```python
from build123d import *

# Parameters (mm, degrees)
SKETCH1_W           = 2.032
SKETCH1_H           = 34.925
BOSS_EXTRUDE1_DEPTH = 228.6
CUT_EXTRUDE1_REACH  = 233.261
SKETCH2_R           = 4.7625
LPATTERN1_COUNT     = 24
LPATTERN1_PITCH     = 19.05
FILLET1_R           = 12.7


with BuildPart() as part:
    # Sketch1 → Boss-Extrude1 (new, symmetric)
    with BuildSketch(Plane.XY):
        with Locations((1.016, 17.4625)):
            Rectangle(SKETCH1_W, SKETCH1_H)
    extrude(amount=BOSS_EXTRUDE1_DEPTH, both=True)

    # Sketch2 → Cut-Extrude1 (cut, up to next)
    with BuildSketch(Plane.ZY, mode=Mode.PRIVATE) as cut_extrude1_sk1:
        with Locations((219.075, 17.4625)):
            Circle(SKETCH2_R)
    cut_extrude1_tool1 = extrude(cut_extrude1_sk1.sketch, amount=-CUT_EXTRUDE1_REACH, mode=Mode.PRIVATE) & part.part
    cut_extrude1 = cut_extrude1_tool1.solids().sort_by_distance((0, 17.4625, 219.075))[0]
    add(cut_extrude1, mode=Mode.SUBTRACT)

    # LPattern1: Cut-Extrude1 ×24
    with Locations(*[(0, 0, -i * LPATTERN1_PITCH) for i in range(1, LPATTERN1_COUNT)]):
        add(cut_extrude1, mode=Mode.SUBTRACT)

    # Fillet1
    fillet1_edges = [part.edges().sort_by_distance(p)[0] for p in [
        (1.016, 34.925, 228.6),
        (1.016, 34.925, -228.6),
        (1.016, 0, -228.6),
        (1.016, 0, 228.6),
    ]]
    fillet(fillet1_edges, radius=FILLET1_R)


solid = part.part
```
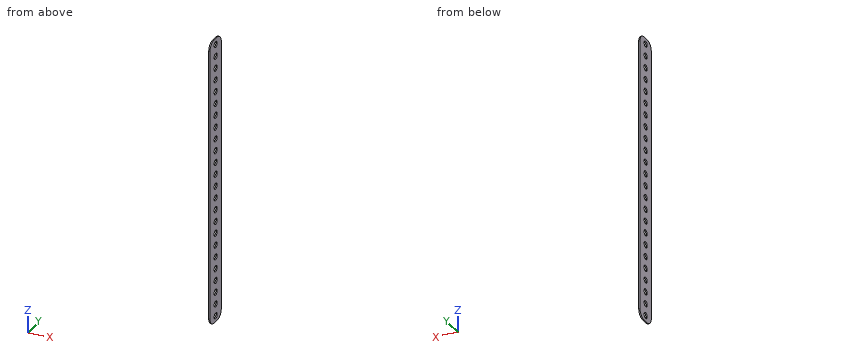
Work out the finished part from the listing and answer in its coordinate system (mm). Give positions to 0.01 mm unless a question says otherwise; leave off trailing zeros. Order: outer loops, then holes, each group sorted by start corner. A loop starts at its lowest first (then second) coordinate and runs counter-clockwise, first axis right, second up. Notation, with made-up numbers: M 20,0.5 L 70,0.5 A29 ccw 70,20.5 Z; hole C 2.5,-34 d11. An arc over 180 degrees is marked long. Return JSON: item names as keys, results as strings.
1) Straight lines are drawn through the part: line 1 along Y through (x, z) = (1.7, 66.5) (3 decimals); line 2 along Y through (x, z) = (0.15, -85) (1 decimal); line 3 along Z through (x, y) = (1.85, 23.5). For each, find the intervals that lie inside material, in ascending order. Write a range as [from, to].
Resolved:
{"line 1": "[0, 12.703], [22.222, 34.925]", "line 2": "[0, 12.8], [22.2, 34.9]", "line 3": "[-228.54, 228.54]"}
2) Section C-C, the plane y = 4 is taken. Write down the section's boundary in (x, z).
Resolved:
{"outline": "M 0,-225.15 L 2.03,-225.15 L 2.03,225.15 L 0,225.15 Z"}
3) Section A-A, the plane z = 48.5 is taken. Write down the section's boundary in (x, y) (3 decimals).
Resolved:
{"outline": "M 0,0 L 2.032,0 L 2.032,12.781 L 0,12.781 Z; M 0,22.144 L 2.032,22.144 L 2.032,34.925 L 0,34.925 Z"}
4) Section D-D, the plane z = 199.5 is taken. Write down the section's boundary in (x, y) (3 decimals).
Resolved:
{"outline": "M 0,0 L 2.032,0 L 2.032,12.729 L 0,12.729 Z; M 0,22.196 L 2.032,22.196 L 2.032,34.925 L 0,34.925 Z"}
5) Section B-B, the plane x = 1.2 is taken. Give the number of separate pieces and of enclosed holes in the cut face, plus the area to 3 significant figures.
Resolved:
{"separate pieces": "1", "enclosed holes": "24", "area": "14,100 mm^2"}
